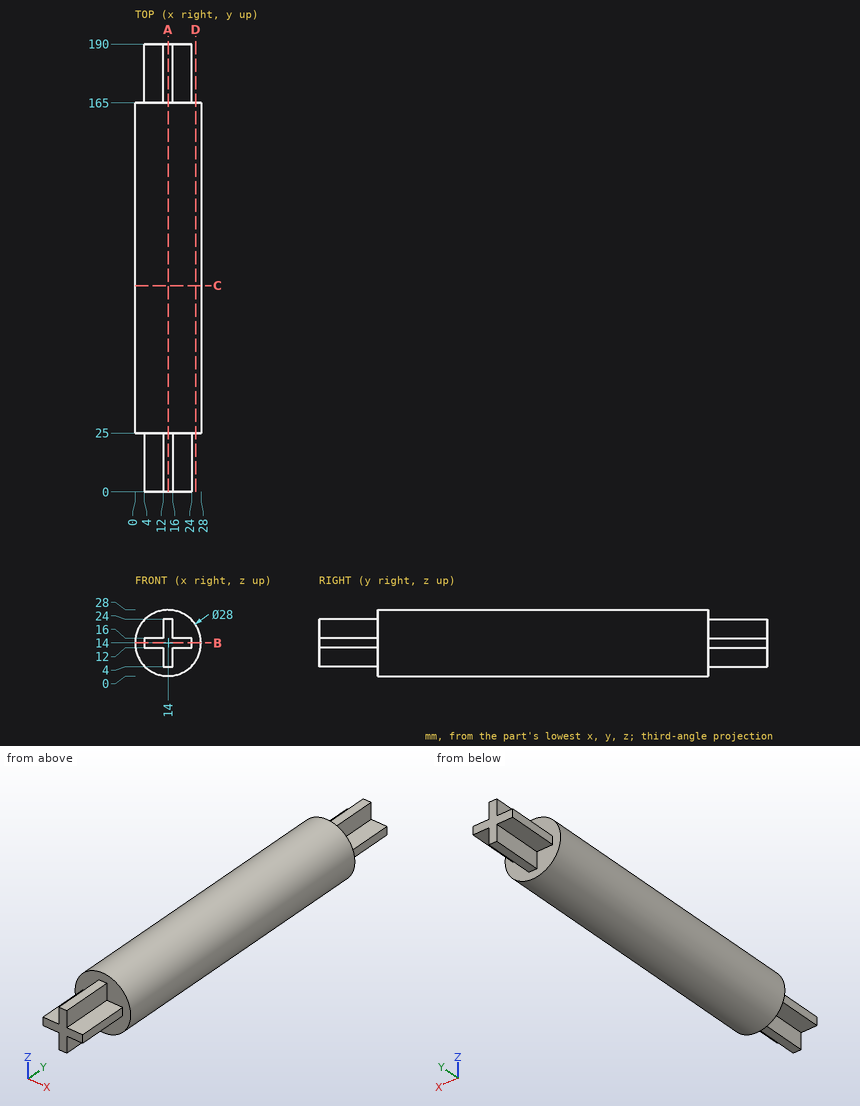
Job drawing, mm, ordinate dimensions from the low corner. One solid piece. Coordinates: 2 decimals unless noted, no trailing zeros. Loops run counter-clockwise (first coordinate to the right, second up) from the corner with the lowest first, then second, coordinate; pieces in that order, holes last. Notation, with made-up numbers: (5, 1.5) - (28, 1.5) arc R27 ccw to (28, 23.5) - close; hole circle Ø8 at (-27, 69.25). An arc over 180 degrees is marked (long way). Answer as a JSON object with one key per item and string values. Group by question number.
(1) Cut at D-D (x = 25.75). Give the cut face in (y, z), then the cut area to 3 significant figures.
(2) Cut at B-B (z = 14). Give the cut face in (x, y), then the cut area to 3 significant figures.
(3) Probe line 1 along Y through (x, z) = (14.75, 2.75); line 2 along X through (y, z) = (181.5, 20). List the from-to ranges inside material, lowest first.
(4) Cut at C-C (y = 87.5). Give the cut face in (x, z).
(5) Cut at A-A (x = 14). Give the cut face in (y, z).
(6) Flat gauge pins, fed straight in: pin 1 (1 mm diameter, centred on x = 24, z = 11, fed in from -Y); pin 2 (3 mm diameter, centred on y = 174.5, z = 13.5, fed in from +X); pin 3 (6.5 mm diameter, centred on x = 7.5, y = 172, fed in from +Z). Where does each tip first touch, or does it go through?
Geometry says:
{
 "1": {"outline": "(25, 6.39) - (165, 6.39) - (165, 21.61) - (25, 21.61) - close", "area": "2,130 mm^2"},
 "2": {"outline": "(0, 25) - (4, 25) - (4, 0) - (24, 0) - (24, 25) - (28, 25) - (28, 165) - (24, 165) - (24, 190) - (4, 190) - (4, 165) - (0, 165) - close", "area": "4,920 mm^2"},
 "3": {"line 1": "y = 25 to 165", "line 2": "x = 12 to 16"},
 "4": {"outline": "circle Ø28 at (14, 14)"},
 "5": {"outline": "(0, 4) - (25, 4) - (25, 0) - (165, 0) - (165, 4) - (190, 4) - (190, 24) - (165, 24) - (165, 28) - (25, 28) - (25, 24) - (0, 24) - close"},
 "6": {"pin 1": "stops at y = 25", "pin 2": "stops at x = 24", "pin 3": "stops at z = 16"}
}
